Verification items for the finished model (mm, model axes). Face numbers are marked on the shaded views. A direction names the side the tool comes from. Give positions to 0.01 mm unless a question says otherwise; leave off trailing zeros. Order: outer loops, then holes, each group sorted by start corner. A loop starts at its lowest first (then second) coordinate and runs counter-clockwise, first axis right, second up. Notation, with made-up numbers: (-3.75, 26) -> (42.25, 26) arc R22 ccw to (42.25, 36) -> close; hole circle Ø5 at (-38, -18.5). An arc over 180 degrees is marked (long way). Return JSON: item names as keys, results as strings. Group by question number.
(1) Cross-section at A-A on x = -78.5. Enter the section's corners in (y, z).
(2) Cross-section at B-B on z = 16.75. State how many separate pieces and enclosed holes the cut face has, then the cut area to 3 significant figures.
(3) Depth check by flat-ended pin: pin 1 Ø5.5 at (x, z) = (-98, 17) entering from -Y; pin 2 Ø6 at (x, z) = (-57, 11.5) entering from -Y; pin 3 Ø3.5 at (x, y) = (-98.92, 10) entering from -Z; pin 4 Ø2 at (x, z) = (-63, 8.5) entering from -Y. Enter the tip coordinate at first touch or a pass-through.
(4) Tool access check on the marked faces 5, 6, 7 and 8. Record the directions out of +Z, -Z, +X, -X, +Y, -Y that give a thin tool (end or side, any length) a straight path to the whole face; none if there is none.
(5) Thickness scan on line 1 along Y through (x, z) = (-98.5, 3.75); line 2 along X through (y, z) = (-12, 14.25); line 3 along Y through (x, z) = (-78, 23.75). Record the ranges inside material, lowest first.
(6) Release check for a two-part mould opening along Y. For the marked faces 1, 2, 3 and 4 record: pulls with the +Y half, pulls with the -Y half, needs draft (parallel to the pull), parting line crosses it, or undercut.
from build123d import *

# Parameters (mm, degrees)
SKETCH2_R           = 3
BOSS_EXTRUDE1_DEPTH = 25
BOSS_EXTRUDE2_DEPTH = 25
SKETCH4_W           = 19.746158687
SKETCH4_H           = 5.000000001
SKETCH4_W_2         = 19.746896681
SKETCH4_H_2         = 5
CUT_EXTRUDE1_DEPTH  = 115.725186296
FILLET1_R           = 2.5
SKETCH5_R           = 3
CUT_EXTRUDE2_DEPTH  = 115.725186296


with BuildPart() as part:
    # Sketch2 → Boss-Extrude1 (new body)
    with BuildSketch(Plane.XY):
        with BuildLine():
            Line((-44.84499572, 33.411675358), (-48.18980095, 39.574873881))
            ThreePointArc((-48.18980095, 39.574873881), (-50.672758106, 41.531314894), (-53.800671062, 41.074261054))
            add(Edge.make_bspline(
                [(-53.800671062, 41.074261054), (-54.48767514, 40.651810622), (-58.202157398, 38.284629617), (-65.057392245, 32.977438932), (-72.95010089, 23.979669569), (-78.627729923, 12.632057233), (-80.687458565, 0.00103574), (-78.627967037, -12.630024416), (-72.950551026, -23.977743332), (-64.551684805, -33.55290014), (-57.571999896, -38.752778812), (-53.808586452, -41.068411447), (-53.800589503, -41.073329934)],
                knots=[5.497383927, 5.497383927, 5.497383927, 5.497383927, 5.533297999, 5.694136685, 5.890486225, 6.086835766, 6.283185307, 6.479534848, 6.675884389, 6.87223393, 7.068583471, 7.069001522, 7.069001522, 7.069001522, 7.069001522], degree=3))
            ThreePointArc((-53.800589503, -41.073329934), (-50.672539001, -41.530627312), (-48.189401667, -39.574138156))
            Line((-48.189401667, -39.574138156), (-44.84499572, -33.411675358))
            ThreePointArc((-44.84499572, -33.411675358), (-44.493215778, -30.482399972), (-46.245407837, -28.108747428))
            add(Edge.make_bspline(
                [(-46.245407837, 28.108747428), (-91.360422528, 0), (-46.245407837, -28.108747428)],
                knots=[5.50397375, 5.50397375, 5.50397375, 7.062396864, 7.062396864, 7.062396864], degree=2, weights=[1, 0.711467813, 1]))
            ThreePointArc((-46.245407837, 28.108747428), (-44.493215778, 30.482399972), (-44.84499572, 33.411675358))
        make_face()
        with Locations((-70.923488038, 10)):
            Circle(SKETCH2_R, mode=Mode.SUBTRACT)
        with Locations((-70.923488038, -10)):
            Circle(SKETCH2_R, mode=Mode.SUBTRACT)
    extrude(amount=BOSS_EXTRUDE1_DEPTH)

    # Sketch3 → Boss-Extrude2 (add)
    with BuildSketch(Plane.XY.offset(25)):
        with BuildLine():
            Line((-74.177329351, 21), (-103.926591357, 21))
            Line((-103.926591357, 21), (-103.926591357, -21))
            Line((-103.926591357, -21), (-74.176591357, -21))
            add(Edge.make_bspline(
                [(-74.177329351, 21), (-75.755958039, 18.282076683), (-78.800306246, 11.573755088), (-80.687458565, 0.00103574), (-78.800400628, -11.572472575), (-75.755678045, -18.281470977), (-74.176591357, -21)],
                knots=[5.939840224, 5.939840224, 5.939840224, 5.939840224, 6.086835766, 6.283185307, 6.479534848, 6.626565531, 6.626565531, 6.626565531, 6.626565531], degree=3))
        make_face()
    extrude(amount=-BOSS_EXTRUDE2_DEPTH)

    # Sketch4 → Cut-Extrude1 (cut, through all)
    with BuildSketch(Plane.XY.offset(25)):
        with Locations((-84.050408695, 18.500000001)):
            Rectangle(SKETCH4_W, SKETCH4_H)
        with Locations((-84.050039698, -18.5)):
            Rectangle(SKETCH4_W_2, SKETCH4_H_2)
    extrude(amount=-CUT_EXTRUDE1_DEPTH, mode=Mode.SUBTRACT)

    # Fillet1
    fillet1_edges = [part.edges().sort_by_distance(p)[0] for p in [
        (-93.923488038, 16, 12.5),
        (-93.923488038, 21.000000001, 12.5),
        (-103.926591357, -21, 12.5),
        (-93.923488038, -21, 12.5),
        (-93.923488038, -16, 12.5),
        (-74.176591357, -16, 12.5),
        (-74.176591357, -21, 12.5),
        (-74.177329351, 21, 12.5),
        (-74.177329351, 16, 12.5),
        (-103.926591357, 21, 12.5),
    ]]
    fillet(fillet1_edges, radius=FILLET1_R - 0.0001)  # a hair under: the kernel refuses the full size

    # Sketch5 → Cut-Extrude2 (cut, through all)
    with BuildSketch(Plane.XY.offset(25)):
        with Locations((-98.923488038, 10)):
            Circle(SKETCH5_R)
        with Locations((-98.923488038, -10)):
            Circle(SKETCH5_R)
    extrude(amount=-CUT_EXTRUDE2_DEPTH, mode=Mode.SUBTRACT)


solid = part.part
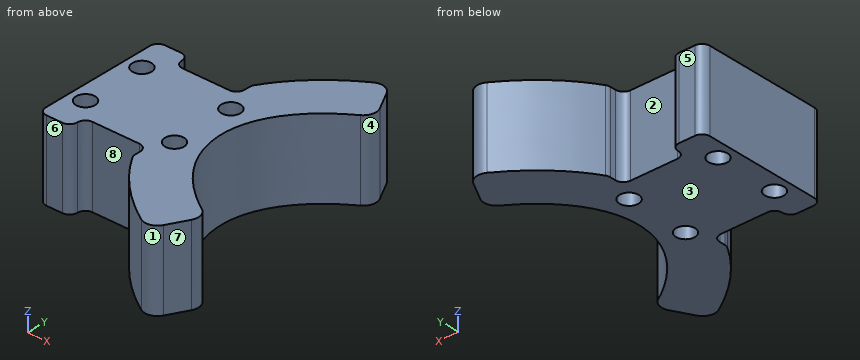
Verdict:
{
 "1": {"outline": "(-16, 0) -> (16, 0) -> (16, 25) -> (-16, 25) -> close"},
 "2": {"separate pieces": "1", "enclosed holes": "4", "area": "2,170 mm²"},
 "3": {"pin 1": "y = -21", "pin 2": "y = -40.95", "pin 3": "through", "pin 4": "y = -35.19"},
 "4": {"face 5": "+Z, -Z, -X, +Y", "face 6": "+Z, -Z, -X, -Y", "face 7": "+Z, -Z, +X, -Y", "face 8": "+Z, -Z, -Y"},
 "5": {"line 1": "-21 to -12.97, -7.03 to 7.03, 12.97 to 21", "line 2": "-103.93 to -101.16, -96.69 to -73.16, -68.69 to -62.01", "line 3": "-16 to 16"},
 "6": {"face 1": "pulls with the -Y half", "face 2": "pulls with the +Y half", "face 3": "needs draft", "face 4": "undercut"}
}
